Read the model definition and answer for the solid it produces. Units are mm, in the model's axes. Give positions to 0.01 mm unless a question says otherwise; leave off trailing zeros. Loops run counter-clockwise (first coordinate to the right, second up) from the corner with the lowest first, then second, coordinate; pieces in that order, holes last. Notation, with made-up numbers: (85.25, 44) - (130.25, 44) arc R24 ccw to (130.25, 66) - close; hole circle Ø5 at (35.5, 74). An arc over 180 degrees is marked (long way). Put each result on its own line as item: value. Start each with the question number.
1. Consider L1, parallel to Y at x = -24, z = 3.05; L2, parallel to Y at x = 12.5, z = 1.4; L3, parallel to Y at x = 24.5, z = 4.15. Determine where each line is inside the solid, lowest interval first. Write a range as from..to.
2. A cutting plane is placed at D-D, the plane y = 0. Determine the outline of the cut face in (x, z), plus the area to 4 significant figures.
3. A cutting plane is placed at C-C, the plane x = -19.5. Determine the outline of the cut face in (y, z), plus the area to 3 significant figures.
4. Given pin 1 Ø1.6 at (y, z) = (28.5, 2) entering from +X; pin 2 Ø1 at (x, z) = (32, 1) entering from +Y; pin 3 Ø3 at (x, z) = (-1, 2) entering from +Y, each flat-ended and moving along its own axis, determine where each tip first touches the part or whether it passes through.
5. A cutting plane is placed at A-A, the plane x = 0. Determine the outline of the cut face in (y, z).
6. A cutting plane is placed at B-B, the plane y = -19.5. Determine the outline of the cut face in (x, z), plus the area to 3 significant figures.
Autodesk Inventor part; units mm, degrees
ref_plane "YZ Plane" through (0, 0, 0) normal (1, 0, 0) x (0, 1, 0)
ref_plane "XZ Plane" through (0, 0, 0) normal (0, 1, 0) x (-1, 0, 0)
ref_plane "XY Plane" through (0, 0, 0) normal (0, 0, 1) x (1, 0, 0)
sketch "Sketch1" plane through (0, 0, 0) normal (0, 0, 1) x (1, 0, 0)
  circle A0 centre (0, 0) radius 54.5
  line L0 (15, 2.8) -> (35, 2.8)
  line L1 (35, 2.8) -> (35, -2.7)
  line L2 (35, -2.7) -> (15, -2.7)
  line L3 (15, -2.7) -> (15, 2.8)
  line L4 (8.6974, 12.6158) -> (22.8395, 26.7579)
  line L5 (22.8395, 26.7579) -> (26.7286, 22.8688)
  line L6 (26.7286, 22.8688) -> (12.5865, 8.7267)
  line L7 (12.5865, 8.7267) -> (8.6974, 12.6158)
  line L8 (-2.7, 15.1) -> (-2.7, 35.1)
  line L9 (-2.7, 35.1) -> (2.8, 35.1)
  line L10 (2.8, 35.1) -> (2.8, 15.1)
  line L11 (2.8, 15.1) -> (-2.7, 15.1)
  line L12 (-12.5158, 8.7974) -> (-26.6579, 22.9395)
  line L13 (-26.6579, 22.9395) -> (-22.7688, 26.8286)
  line L14 (-22.7688, 26.8286) -> (-8.6267, 12.6865)
  line L15 (-8.6267, 12.6865) -> (-12.5158, 8.7974)
  line L16 (-15, -2.6) -> (-35, -2.6)
  line L17 (-35, -2.6) -> (-35, 2.9)
  line L18 (-35, 2.9) -> (-15, 2.9)
  line L19 (-15, 2.9) -> (-15, -2.6)
  line L20 (-8.6974, -12.4158) -> (-22.8395, -26.5579)
  line L21 (-22.8395, -26.5579) -> (-26.7286, -22.6688)
  line L22 (-26.7286, -22.6688) -> (-12.5865, -8.5267)
  line L23 (-12.5865, -8.5267) -> (-8.6974, -12.4158)
  line L24 (2.7, -14.9) -> (2.7, -34.9)
  line L25 (2.7, -34.9) -> (-2.8, -34.9)
  line L26 (-2.8, -34.9) -> (-2.8, -14.9)
  line L27 (-2.8, -14.9) -> (2.7, -14.9)
  line L28 (12.5158, -8.5974) -> (26.6579, -22.7395)
  line L29 (26.6579, -22.7395) -> (22.7688, -26.6286)
  line L30 (22.7688, -26.6286) -> (8.6267, -12.4865)
  line L31 (8.6267, -12.4865) -> (12.5158, -8.5974)
  line L32 (24.2998, 0.05) -> (27.4417, 0.05)
  point P0 (0, 0.1)
  dimension "d0" = 109
  dimension "d3" = 20
  dimension "d4" = 5.5
  dimension "d5" = 360
  dimension "d8" = 2.75
extrude "Extrusion1" add sketch "Sketch1" along normal blind 5.5
properties part number "medio"
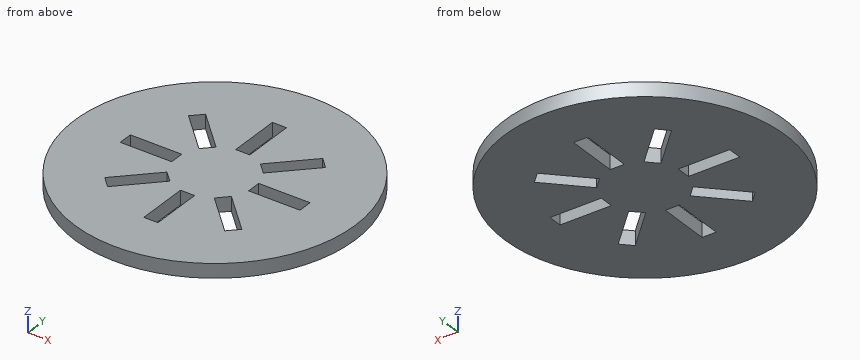
Return value:
1. L1: y = -48.93..-25.4, -19.94..-2.6, 2.9..20.28, 25.6..48.93
1. L2: y = -53.05..-16.36, -8.61..8.81, 16.42..53.05
1. L3: y = -48.68..-24.9, -20.58..-2.7, 2.8..20.64, 25.1..48.68
2. outline: (-54.5, 0) - (-35, 0) - (-35, 5.5) - (-54.5, 5.5) - close; (-15, 0) - (15, 0) - (15, 5.5) - (-15, 5.5) - close; (35, 0) - (54.5, 0) - (54.5, 5.5) - (35, 5.5) - close
2. area: 379.5 mm2
3. outline: (-50.89, 0) - (-23.22, 0) - (-23.22, 5.5) - (-50.89, 5.5) - close; (-15.44, 0) - (-2.6, 0) - (-2.6, 5.5) - (-15.44, 5.5) - close; (2.9, 0) - (15.78, 0) - (15.78, 5.5) - (2.9, 5.5) - close; (23.56, 0) - (50.89, 0) - (50.89, 5.5) - (23.56, 5.5) - close
3. area: 444 mm2
4. pin 1: stops at x = 46.94
4. pin 2: stops at y = 44.47
4. pin 3: stops at y = 54.5
5. outline: (-54.5, 0) - (-34.9, 0) - (-34.9, 5.5) - (-54.5, 5.5) - close; (-14.9, 0) - (15.1, 0) - (15.1, 5.5) - (-14.9, 5.5) - close; (35.1, 0) - (54.5, 0) - (54.5, 5.5) - (35.1, 5.5) - close
6. outline: (-50.89, 0) - (-23.56, 0) - (-23.56, 5.5) - (-50.89, 5.5) - close; (-15.78, 0) - (-2.8, 0) - (-2.8, 5.5) - (-15.78, 5.5) - close; (2.7, 0) - (15.64, 0) - (15.64, 5.5) - (2.7, 5.5) - close; (23.42, 0) - (50.89, 0) - (50.89, 5.5) - (23.42, 5.5) - close
6. area: 444 mm2
